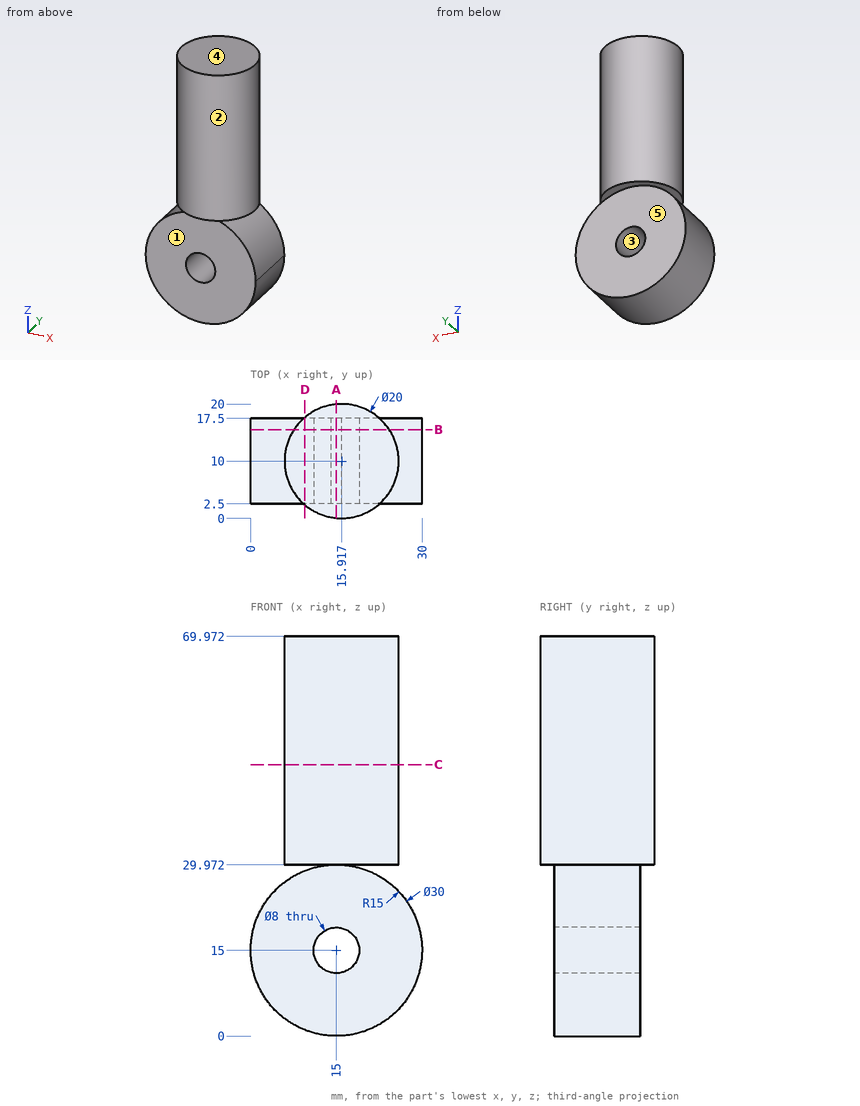
Input: dimensioned drawing with shaded views. Units: mm. Origin: part minimum x, y, z. A direction names the side the tool comes from. Coordinates: 2 decimals unless noted, no trailing zeros. Loops run counter-clockwise (first coordinate to the right, second up) from the corner with the lowest first, then second, coordinate; pieces in that order, holes last. Notation, with made-up numbers: (-1.75, 13) -> (48.25, 13) arc R28 ccw to (48.25, 43) -> close; hole circle Ø8 at (17.5, -26). An arc over 180 degrees is marked (long way). Use a Markdown table: item, result. Add a question column.
(1) Mould query, pull axis Z, two halves, no side actions, for the marked faces 3, 4 and 5. Classes: pulls with the +Z half, pulls with the -Z half, needs draft (parallel to the pull), parting line crosses it, or undercut.
(2) Pin query (flat end, axial travel): pin 1 Ø1 at (x, y) = (7, 13.5) entering from -Z; pin 2 Ø1 at (y, z) = (10.5, 60.5) entering from +X; pin 3 Ø6 at (x, z) = (11.5, 16.5) entering from -Y; pin 4 Ø7 at (x, z) = (15, 15) entering from -Y. Return the tip coordinate at first contact, or that it passes through.
(3) Section query B-B, the plane y = 15.5. Return loops of the section in (x, z).
(4) Access query for the marked faces 1 and 2. Directions: +Z, -Z, +X, -X, +Y, -Y. A direction counts if a zero-diameter tool reaches every point of the face in a straight line with its end or side. Return the directions, or none.
(5) Section query D-D, the plane x = 9.5. Return loops of the section in (y, z) (1 decimal), plus the area to 3 significant figures.
(6) Section query C-C, the plane z = 47.5. Return loops of the section in (x, y).
(7) Line query: line 1 along X through (y, z) = (12.5, 15); line 2 along Z through (x, y) = (15, 10.5); line 3 along Y through (x, z) = (15.75, 61). Output: solid intervals per line, ascending.
(8) Section query A-A, the plane x = 15. Return loops of the section in (y, z), plus the area to 3 significant figures.
Answer:
| question | item | result |
|---|---|---|
| 1 | face 3 | undercut |
| 1 | face 4 | pulls with the +Z half |
| 1 | face 5 | needs draft |
| 2 | pin 1 | stops at z = 2.01 |
| 2 | pin 2 | stops at x = 25.92 |
| 2 | pin 3 | stops at y = 2.5 |
| 2 | pin 4 | passes through |
| 3 | outline | (7.57, 29.97) -> (14.08, 29.97) arc R15 ccw (long way) to (15.92, 29.97) -> (24.27, 29.97) -> (24.27, 69.97) -> (7.57, 69.97) -> close; hole circle Ø8 at (15, 15) |
| 4 | face 1 | -Z, +X, -X, -Y |
| 4 | face 2 | +Z |
| 5 | outline | (2.3, 30) -> (17.7, 30) -> (17.7, 70) -> (2.3, 70) -> close; (2.5, 1) -> (17.5, 1) -> (17.5, 29) -> (2.5, 29) -> close |
| 5 | area | 1,030 mm^2 |
| 6 | outline | circle Ø20 at (15.92, 10) |
| 7 | line 1 | x = 0 to 11, 19 to 30 |
| 7 | line 2 | z = 0 to 11, 19 to 69.97 |
| 7 | line 3 | y = 0 to 20 |
| 8 | outline | (0.04, 29.97) -> (2.5, 29.97) -> (2.5, 19) -> (17.5, 19) -> (17.5, 29.97) -> (19.96, 29.97) -> (19.96, 69.97) -> (0.04, 69.97) -> close; (2.5, 0) -> (17.5, 0) -> (17.5, 11) -> (2.5, 11) -> close |
| 8 | area | 1,130 mm^2 |
